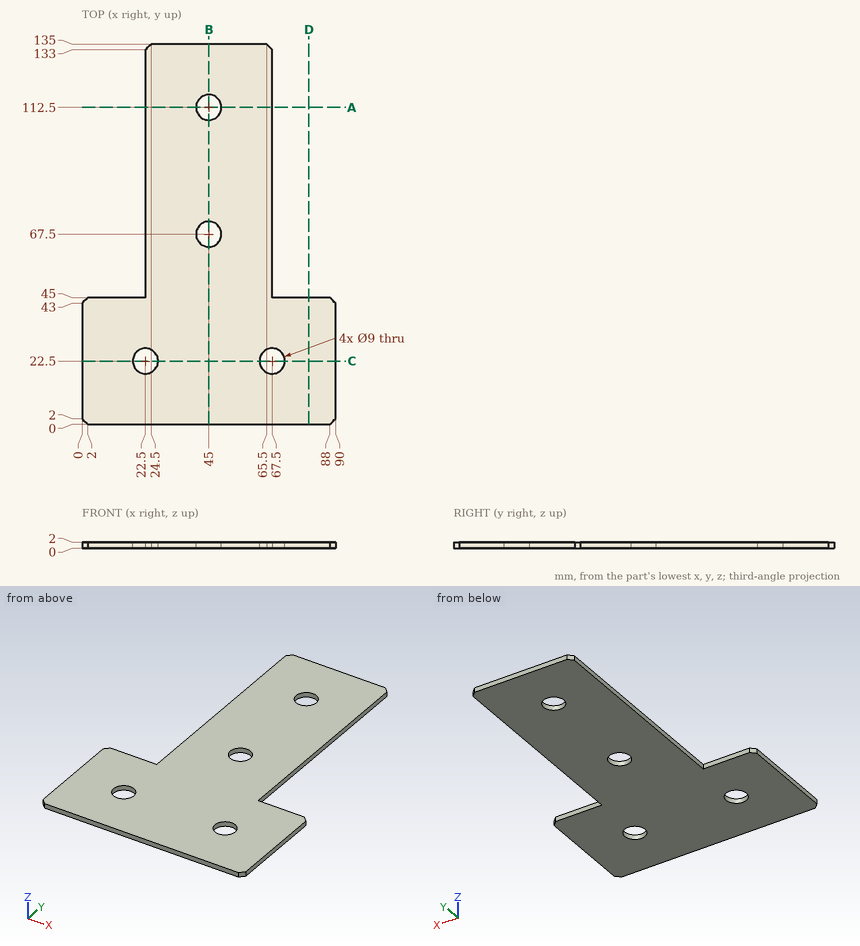
Job drawing, mm, ordinate dimensions from the low corner. One solid piece. Coordinates: 2 decimals unless noted, no trailing zeros. Write each loop counter-clockwise with the first axis right and the second up, starting at its lowest first coordinate (ties: lowest second). Pieces come first, ordered by that corner, then holes. Notation, with made-up numbers: (-33, 25.25) - (2, 25.25) arc R12 cw to (2, 46.25) - close; hole circle Ø7 at (73, -39). An arc over 180 degrees is marked (long way). Use a Markdown table: item, result. Add a question column.
Item 1: Flat gauge pins, fed straight in: pin 1 (8 mm diameter, centred on x = 67.5, y = 22.5, fed in from +Z); pin 2 (1 mm diameter, centred on y = 103, z = 1, fed in from +X); pin 3 (1 mm diameter, centred on y = 97.5, z = 0.5, fed in from -X). Where does each tip first touch, or does it go through?
Item 2: Band-saw the part on A-A, the plane y = 112.5. Give the cut face in (x, z), and give its area (3 significant figures).
Item 3: Band-saw the part on B-B, the plane x = 45. Give the cut face in (y, z).
Item 4: Band-saw the part on D-D, the plane x = 80.5. Give the cut face in (y, z).
Item 5: Drill centre lines: L1, parallel to Y at x = 45, z = 0.55; L2, parallel to X at y = 22.5, z = 1.05; L3, parallel to X at y = 112.5, z = 0.8. Where is each one in solid material? Low to high. Write a range as from..to.
Item 6: Band-saw the part on C-C, the plane y = 22.5. Give the cut face in (x, z).
Numbers:
| question | item | result |
|---|---|---|
| 1 | pin 1 | through |
| 1 | pin 2 | x = 67.5 |
| 1 | pin 3 | x = 22.5 |
| 2 | outline | (22.5, 0) - (40.5, 0) - (40.5, 2) - (22.5, 2) - close; (49.5, 0) - (67.5, 0) - (67.5, 2) - (49.5, 2) - close |
| 2 | area | 72.0 mm2 |
| 3 | outline | (0, 0) - (63, 0) - (63, 2) - (0, 2) - close; (72, 0) - (108, 0) - (108, 2) - (72, 2) - close; (117, 0) - (135, 0) - (135, 2) - (117, 2) - close |
| 4 | outline | (0, 0) - (45, 0) - (45, 2) - (0, 2) - close |
| 5 | L1 | 0..63, 72..108, 117..135 |
| 5 | L2 | 0..18, 27..63, 72..90 |
| 5 | L3 | 22.5..40.5, 49.5..67.5 |
| 6 | outline | (0, 0) - (18, 0) - (18, 2) - (0, 2) - close; (27, 0) - (63, 0) - (63, 2) - (27, 2) - close; (72, 0) - (90, 0) - (90, 2) - (72, 2) - close |
